Geometry: final body of the model. Coordinates: model frame, mm. Round coordinates to 2 decimals unless told otherwise and drop trailing zeros. Loops run counter-clockwise (first coordinate to the right, second up) from the corner with the lowest first, then second, coordinate; pieces in that order, holes last. Notation, with made-up numbers: (21, -2.5) -> (44, -2.5) arc R33 ccw to (44, 26.5) -> close; hole circle Ø6 at (6.5, -26). An arc over 180 degrees is marked (long way). Answer in a Markdown table with one row per item.
```python
from build123d import *

# Parameters (mm, degrees)
F1_DEPTH = 25
F3_D     = 2.5
F5_R     = 12.8012424822
F5_R_2   = 2.45
F6_DEPTH = 19


with BuildPart() as f1:
    # F0 (on Top) → F1 (new body)
    with BuildSketch(Plane.XY):
        Polygon((1.643359007, -2.3733319421), (2.877045257, 0.2365246766), (1.2336862499, 2.6098566187), (-1.643359007, 2.3733319421), (-2.877045257, -0.2365246766), (-1.2336862499, -2.6098566187), align=None)
    extrude(amount=F1_DEPTH)

    # F3 (through all)
    with Locations(Plane.XY.offset(25)):
        with Locations((0, 0)):
            Hole(F3_D / 2)


with BuildPart() as f6:
    # F5 (on offset) → F6 (new body)
    with BuildSketch(Plane.XY.offset(3)):
        Circle(F5_R)
        Circle(F5_R_2, mode=Mode.SUBTRACT)
    extrude(amount=F6_DEPTH)


with BuildPart() as f1_1:
    add(f1.part)

    # F7: cut F6
    add(f6.part, mode=Mode.SUBTRACT)


solid = f1_1.part
```
Item 1: Section query C-C, the plane z = 10. Output: boundary loops of the cut face in (x, y), and give its area (3 significant figures).
Ans:
| item | result |
|---|---|
| outline | circle Ø4.9 at (0, 0); hole circle Ø2.5 at (0, 0) |
| area | 13.9 mm2 |
Item 2: Mould query, pull axis Z, two halves, no side actions, for faces 1 (the flat face through (1, -1, 25)), 2 (the flat face through (2.25, -1.09, 1.48)), 3 (the cylindrical face through (-0.5, -2.4, 12.4)), 4 (the flat face through (1, -1, 0)). Classes: released by +Z, released by -Z, zero draft, split by the parting line, or undercut.
Ans:
| item | result |
|---|---|
| face 1 | released by +Z |
| face 2 | zero draft |
| face 3 | undercut |
| face 4 | released by -Z |
Item 3: Section query D-D, the plane y = 1.6. Output: boundary loops of the cut face in (x, z).
Ans:
| item | result |
|---|---|
| outline | (-2.01, 0) -> (1.93, 0) -> (1.93, 3) -> (1.86, 3) -> (1.86, 22) -> (1.93, 22) -> (1.93, 25) -> (-2.01, 25) -> (-2.01, 22) -> (-1.86, 22) -> (-1.86, 3) -> (-2.01, 3) -> close |
Item 4: Section query A-A, the plane x = 0. Output: boundary loops of the cut face in (y, z).
Ans:
| item | result |
|---|---|
| outline | (-2.51, 0) -> (-1.25, 0) -> (-1.25, 25) -> (-2.51, 25) -> (-2.51, 22) -> (-2.45, 22) -> (-2.45, 3) -> (-2.51, 3) -> close; (1.25, 0) -> (2.51, 0) -> (2.51, 3) -> (2.45, 3) -> (2.45, 22) -> (2.51, 22) -> (2.51, 25) -> (1.25, 25) -> close |
Item 5: Ray query, L1, parallel to Y at x = 0, z = 5.5; L2, parallel to Y at x = 1, z = 12.5; L3, parallel to X at y = -0.4, z = 23.75. Return the intervals inside material, ascending.
Ans:
| item | result |
|---|---|
| L1 | -2.45 to -1.25, 1.25 to 2.45 |
| L2 | -2.24 to -0.75, 0.75 to 2.24 |
| L3 | -2.76 to -1.18, 1.18 to 2.58 |
Item 6: Section query B-B, the plane y = 0. Output: boundary loops of the cut face in (x, z), and give its area (3 significant figures).
Ans:
| item | result |
|---|---|
| outline | (-2.77, 0) -> (-1.25, 0) -> (-1.25, 25) -> (-2.77, 25) -> (-2.77, 22) -> (-2.45, 22) -> (-2.45, 3) -> (-2.77, 3) -> close; (1.25, 0) -> (2.77, 0) -> (2.77, 3) -> (2.45, 3) -> (2.45, 22) -> (2.77, 22) -> (2.77, 25) -> (1.25, 25) -> close |
| area | 63.8 mm2 |
Item 7: First-contact query: P1, Ø2, axis at x = 0, z = 17.5, coming from the -Y side. Flat tip, straight axial feed; report the tip coordinate or a pass-through.
Ans:
| item | result |
|---|---|
| P1 | y = -2.45 |
